Geometry check sheet. Reference: the model listing, model coordinates, mm. Face numbers are marked on the shaded views. A direction names the side the tool comes from. Round coordinates to 2 decimals unless told otherwise and drop trailing zeros. Write each loop counter-clockwise with the first axis right and the second up, starting at its lowest first coordinate (ties: lowest second). Pieces come first, ordered by that corner, then holes.
from build123d import *

# Parameters (mm, degrees)
F0_R     = 2.3114
F1_DEPTH = 12.7
F2_R     = 2.3114
F3_DEPTH = 25.4
F4_R     = 2.3114
F5_DEPTH = 3.81


with BuildPart() as f1:
    # F0 (on Front) → F1 (new body)
    with BuildSketch(Plane.XZ):
        Polygon((0, 25.4), (0, 0), (25.4, 0), (25.4, 3.81), (12.7, 3.81), (12.7, 25.4), align=None)
        with Locations((6.35, 6.35)):
            Circle(F0_R, mode=Mode.SUBTRACT)
    extrude(amount=F1_DEPTH)

    # F2 (on face) → F3 (cut)
    with BuildSketch(Plane(origin=(0, 0, 0), x_dir=(0, -1, 0), z_dir=(-1, 0, 0))):
        with Locations((6.35, 19.05)):
            Circle(F2_R)
    extrude(amount=-F3_DEPTH, mode=Mode.SUBTRACT)

    # F4 (on face) → F5 (cut)
    with BuildSketch(Plane.XY.offset(3.81)):
        with Locations((19.05, -6.35)):
            Circle(F4_R)
    extrude(amount=-F5_DEPTH, mode=Mode.SUBTRACT)


solid = f1.part
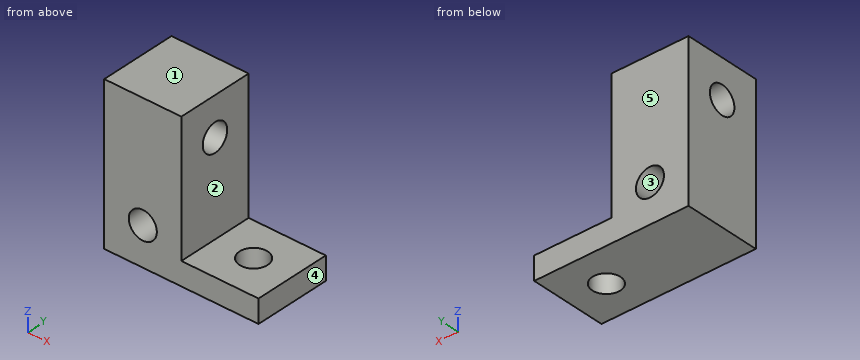
1. Section check D-D (x = 19.05). Record the cut outline in (y, z).
2. Release check for a two-part mould opening along X. For the marked faces 3, 4 and 5 record: +X half, -X half, draft (parallel to the pull), parting line (faces both ways), or undercut.
3. Section check A-A (x = 6.35). Record the cut outline in (y, z).
4. Scan lines: line 1 along Z through (x, y) = (9.25, -6.35); line 2 along Z through (x, y) = (6.35, -9); line 3 along Z through (x, y) = (6.25, -7.75). Record each from-to range of solid material in increasing order.
5. Section check C-C (z = 19.05). Record the cut outline in (x, y), plus the area to 3 significant figures.
6. Access from +Z, -Z, +X, -X, +Y, -Y to the whole of each face (thin tool, end or side, straight path). Record for the marked faces 1 and 2.
7. Depth check by flat-ended pin: pin 1 Ø7.5 at (y, z) = (-6.35, 19.05) entering from +X; pin 2 Ø1 at (x, y) = (4.5, -10) entering from -Z. Enter the tip coordinate at first touch or a pass-through.
8. Section check B-B (y = -6.35). Record the cut outline in (x, z).
Results below:
1. outline: (-12.7, 0) - (-8.66, 0) - (-8.66, 3.81) - (-12.7, 3.81) - close; (-4.04, 0) - (0, 0) - (0, 3.81) - (-4.04, 3.81) - close
2. face 3: undercut
2. face 4: +X half
2. face 5: draft
3. outline: (-12.7, 0) - (0, 0) - (0, 4.04) - (-12.7, 4.04) - close; (-12.7, 8.66) - (0, 8.66) - (0, 25.4) - (-12.7, 25.4) - close; hole circle Ø4.62 at (-6.35, 19.05)
4. line 1: z = 0 to 16.74, 21.36 to 25.4
4. line 2: z = 0 to 4.04, 8.66 to 25.4
4. line 3: z = 0 to 4.04, 8.66 to 17.21, 20.89 to 25.4
5. outline: (0, -12.7) - (12.7, -12.7) - (12.7, -8.66) - (0, -8.66) - close; (0, -4.04) - (12.7, -4.04) - (12.7, 0) - (0, 0) - close
5. area: 103 mm2
6. face 1: +Z, +X, -X, +Y, -Y
6. face 2: +Z, +X, +Y, -Y
7. pin 1: stops at x = 12.7
7. pin 2: stops at z = 0
8. outline: (0, 0) - (16.74, 0) - (16.74, 3.81) - (12.7, 3.81) - (12.7, 16.74) - (0, 16.74) - close; (0, 21.36) - (12.7, 21.36) - (12.7, 25.4) - (0, 25.4) - close; (21.36, 0) - (25.4, 0) - (25.4, 3.81) - (21.36, 3.81) - close; hole circle Ø4.62 at (6.35, 6.35)
